Input: dimensioned drawing with shaded views. Units: mm. Origin: part minimum x, y, z. A direction names the side the tool comes from. Round coordinates to 2 decimals unless told otherwise and drop trailing zeros. Loops run counter-clockwise (first coordinate to the right, second up) from the corner with the lowest first, then second, coordinate; pieces in that order, holes last. Notation, with made-up numbers: M 40.5,85.5 L 80.5,85.5 A28 ccw 80.5,122.5 Z; hole C 89.25,34.25 d5. An arc over 180 degrees is marked long. Write each question's results on one line, items separated by ' | '. Start each with the question number.
1. Ray query, line 1 (X direction, y = 80, z = 38); line 2 (Z direction, x = 3, y = 78); line 3 (Y direction, x = 11.25, z = 68). Return the intervals inside material, ascending.
2. Section C-C on y = 10. Output: boundary loops of the cut face in (x, z).
3. Section A-A on y = 78. Output: boundary loops of the cut face in (x, z), and give its area (3 significant figures).
4. Section D-D on z = 15. Output: boundary loops of the cut face in (x, y), and give its area (3 significant figures).
5. Contact query for flat-ended pins moving along their axis: pin 1 Ø8.5 at (y, z) = (11, 8.5) entering from -X; pin 2 Ø17.5 at (x, z) = (5, 46.5) entering from -Y; pin 3 Ø16 at (x, y) = (39, 11) entering from +Z; pin 4 Ø10 at (x, y) = (50, 35) entering from +Z. Output: stop coordinate, or through.
6. Set-up query: the marked faces 1, 2, 3, 4 and 5. Return all of +Z, -Z, +X, -X, +Y, -Y with unobstructed straight access to the full face (end or side cutting, diameter ignored); none if empty.
7. Draft query along X for the marked faces 6, 7, 8 and 9. Return one class per face: released by +X, released by -X, zero draft, split by the parting line, or undercut.
8. Section B-B on x = 67.5. Output: boundary loops of the cut face in (y, z).
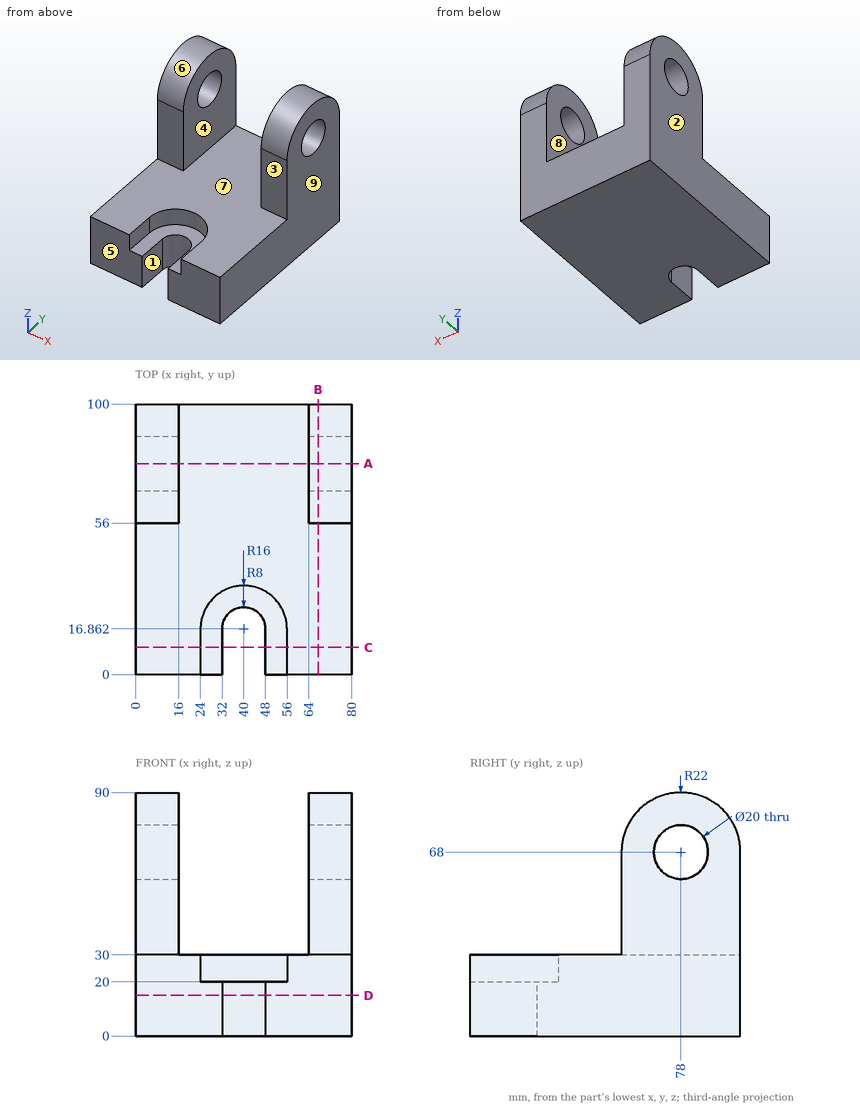
Taken from the geometry:
1) line 1: 0 to 16, 64 to 80 | line 2: 0 to 58, 78 to 90 | line 3: 56 to 68, 88 to 100
2) outline: M 0,0 L 32,0 L 32,20 L 24,20 L 24,30 L 0,30 Z; M 48,0 L 80,0 L 80,30 L 56,30 L 56,20 L 48,20 Z
3) outline: M 0,0 L 80,0 L 80,58 L 64,58 L 64,30 L 16,30 L 16,58 L 0,58 Z; M 0,78 L 16,78 L 16,90 L 0,90 Z; M 64,78 L 80,78 L 80,90 L 64,90 Z | area: 3,680 mm^2
4) outline: M 0,0 L 32,0 L 32,16.86 A8 cw 48,16.86 L 48,0 L 80,0 L 80,100 L 0,100 Z | area: 7,630 mm^2
5) pin 1: x = 0 | pin 2: y = 56 | pin 3: z = 20 | pin 4: z = 30
6) face 1: +Z, -Z, -Y | face 2: +Z, -Z, -X, +Y, -Y | face 3: +Z, +X, -X, -Y | face 4: +Z, +Y, -Y | face 5: +Z, -Z, +X, -X, -Y
7) face 6: zero draft | face 7: undercut | face 8: undercut | face 9: released by +X
8) outline: M 0,0 L 100,0 L 100,68 A22 ccw 56,68 L 56,30 L 0,30 Z; hole C 78,68 d20
